Verification items for the finished model (mm, model axes). A direction names the side the tool comes from. Round coordinates to 2 decimals unless told otherwise and drop trailing zeros. Loops run counter-clockwise (first coordinate to the right, second up) from the corner with the lowest first, then second, coordinate; pieces in that order, holes last. Notation, with made-up numbers: (4, -32.75) -> (55, -32.75) arc R23 cw to (55, -23.75) -> close; hole circle Ø7 at (19.5, 46.5). An arc over 180 degrees is marked (long way). Write item = value, one per line.
```python
from build123d import *

# Parameters (mm, degrees)
SKETCH1_W           = 117
SKETCH1_H           = 117
BOSS_EXTRUDE1_DEPTH = 40
SKETCH2_W           = 10.53028371
SKETCH2_H           = 7.9375
CUT_EXTRUDE1_DEPTH  = 12.7
SKETCH7_W           = 7
SKETCH7_H           = 1.5
CUT_EXTRUDE5_DEPTH  = 41
CIRPATTERN3_COUNT   = 3
CIRPATTERN3_ANGLE   = 180
CUT_EXTRUDE11_DEPTH = 41


with BuildPart() as part:
    # Sketch1 → Boss-Extrude1 (new body)
    with BuildSketch(Plane(origin=(0, 0, 0), x_dir=(1, 0, 0), z_dir=(0, 1, 0))):
        with Locations((58.5, 58.5)):
            Rectangle(SKETCH1_W, SKETCH1_H)
    extrude(amount=BOSS_EXTRUDE1_DEPTH)

    # Sketch2 → Cut-Extrude1 (cut)
    with BuildSketch(Plane(origin=(0, 40, 0), x_dir=(1, 0, 0), z_dir=(0, 1, 0))):
        with BuildLine():
            ThreePointArc((63.765141855, 66.4375), (66.892737967, 63.004173), (68.025, 58.5))
            Line((68.025, 58.5), (68.025, 74.375))
            Line((68.025, 74.375), (48.975, 74.375))
            Line((48.975, 74.375), (48.975, 58.5))
            ThreePointArc((48.975, 58.5), (50.107262033, 63.004173), (53.234858145, 66.4375))
            ThreePointArc((53.234858145, 66.4375), (58.5, 68.025), (63.765141855, 66.4375))
        make_face()
        with BuildLine():
            ThreePointArc((63.765141855, 50.5625), (66.892737967, 53.995827), (68.025, 58.5))
            Line((68.025, 58.5), (63.765141855, 58.5))
            Line((63.765141855, 58.5), (63.765141855, 50.5625))
        make_face()
        with BuildLine():
            Line((63.765141855, 58.5), (68.025, 58.5))
            ThreePointArc((68.025, 58.5), (66.892737967, 63.004173), (63.765141855, 66.4375))
            Line((63.765141855, 66.4375), (63.765141855, 58.5))
        make_face()
        with BuildLine():
            Line((53.234858145, 50.5625), (53.234858145, 58.5))
            Line((53.234858145, 58.5), (48.975, 58.5))
            ThreePointArc((48.975, 58.5), (50.107262033, 53.995827), (53.234858145, 50.5625))
        make_face()
        with BuildLine():
            Line((48.975, 58.5), (53.234858145, 58.5))
            Line((53.234858145, 58.5), (53.234858145, 66.4375))
            ThreePointArc((53.234858145, 66.4375), (50.107262033, 63.004173), (48.975, 58.5))
        make_face()
        with Locations((58.5, 62.46875)):
            Rectangle(SKETCH2_W, SKETCH2_H)
        with BuildLine():
            Line((53.234858145, 66.4375), (63.765141855, 66.4375))
            ThreePointArc((63.765141855, 66.4375), (58.5, 68.025), (53.234858145, 66.4375))
        make_face()
        with Locations((58.5, 54.53125)):
            Rectangle(SKETCH2_W, SKETCH2_H)
    extrude(amount=-CUT_EXTRUDE1_DEPTH, mode=Mode.SUBTRACT)

    # Sketch7 → Cut-Extrude5 (cut, through all)
    with BuildSketch(Plane.XZ):
        with Locations((58.5, -117)):
            Rectangle(SKETCH7_W, SKETCH7_H)
    cut_extrude5 = extrude(amount=-CUT_EXTRUDE5_DEPTH, mode=Mode.SUBTRACT)

    # CirPattern3: Cut-Extrude5 ×3 about axis
    cirpattern3_axis = Axis((58.5, 0, -58.5), (0, -1, 0))
    for i in range(1, CIRPATTERN3_COUNT):
        add(cut_extrude5.rotate(cirpattern3_axis, i * CIRPATTERN3_ANGLE / (CIRPATTERN3_COUNT - 1)), mode=Mode.SUBTRACT)

    # Sketch11 → Cut-Extrude11 (cut, through all)
    with BuildSketch(Plane.XZ):
        Polygon((0, -117), (117, 0), (188.640274668, -71.640274668), (71.640274668, -188.640274668), align=None)
    extrude(amount=-CUT_EXTRUDE11_DEPTH, mode=Mode.SUBTRACT)


solid = part.part
```
(1) Sectioned sample at C-C, the plane x = 109.5. Record the cut outline in (y, z).
Filled sheet:
outline = (0, -7.5) -> (40, -7.5) -> (40, 0) -> (0, 0) -> close
(2) Sectioned sample at A-A, the plane y = 5. Record the cut outline in (x, z).
Filled sheet:
outline = (0, -117) -> (117, 0) -> (62, 0) -> (62, -0.75) -> (55, -0.75) -> (55, 0) -> (0, 0) -> close
(3) Go/stop test with flat-tipped pins: pin 1 Ø8 at (x, z) = (60.5, -60) entering from +Y; pin 2 Ø3 at (x, y) = (60, 36) entering from -Z; pin 3 Ø2 at (x, y) = (95.5, 34) entering from -Z. Record where each tip stops, or that it passes through.
Filled sheet:
pin_1 = 27.3
pin_2 = -50.56
pin_3 = -22.5
(4) Sectioned sample at B-B, the plane z = -45. Record the cut outline in (x, y).
Filled sheet:
outline = (0, 0) -> (72, 0) -> (72, 40) -> (0, 40) -> close
(5) Material ranges on probe 1 along Z at (x, y) = (101, 27); probe 2 along X at (y, z) = (28, -104); probe 3 along Z at (x, y) = (63, 22), recorded low to high. Write a range as from..to.
Filled sheet:
probe_1 = -16..0
probe_2 = 0..13
probe_3 = -54..0
(6) Draft check along X on faces 4 (the face through (58, 20, -59)), 5 (the face through (58, 34, -50.562)), 6 (the face through (89, 20, 0)). Enter one of: released by +X, released by -X, zero draft, split by the parting line, or undercut.
Filled sheet:
face_4 = released by +X
face_5 = undercut
face_6 = zero draft
(7) Set-up check for faces 1 (the face through (48.975, 34, -63)), 2 (the face through (59, 20, -0.75)), 3 (the face through (50.08, 33.74, -54.05)): record each of +Z, -Z, +X, -X, +Y, -Y from which the full face is reachable in a straight line by a thin tool's end or side.
Filled sheet:
face_1 = -Z, +X, +Y
face_2 = +Z, +Y, -Y
face_3 = -Z, +Y
